Verification items for the finished model (mm, model axes). Face numbers are marked on the shaded views. Coordinates: 2 decimals unless noted, no trailing zeros. Order: outer loops, then holes, each group sorted by start corner. A loop starts at its lowest first (then second) coordinate and runs counter-clockwise, first axis right, second up. Notation, with made-up numbers: M 36.25,60 L 93.25,60 A14 ccw 93.25,64 Z; hole C 21.5,-32 d8. An arc over 180 degrees is marked long. Return JSON: item names as keys, results as strings. Group by question number.
Q1. Thickness scan on probe 1 along Y at (x, z) = (0, 68.75); probe 2 along Y at (x, z) = (0, 45.5); probe 3 along Z at (x, y) = (67.5, 74). Record the ranges inside material, lowest first.
Q2. Go/stop test with flat-tipped pins: pin 1 Ø1.5 at (x, z) = (71, 57) entering from +Y; pin 2 Ø0.9 at (y, z) = (-83.5, 5.5) entering from +X; pin 3 Ø10 at (y, z) = (-69, 57.5) entering from -X. Record where each tip stops, or that it passes through.
Q3. Mould release check, pull along Z, two halves, no side actions. Record for the marked faces 1, 2, 3 and 4: pulls with the +Z half, pulls with the -Z half, needs draft (parallel to the pull), parting line crosses it, or undercut.
Q4. Section check A-A, the plane y = 0. Enter the section's corners in (x, z), then the cut area to 3 significant figures.
Q5. Section check C-C, the plane x = -66.5. Enter the section's corners in (y, z).
Q6. Section check D-D, the plane y = 48. Enter the section's corners in (x, z).
from build123d import *

# Parameters (mm, degrees)
SKETCH1_R           = 100.8
SKETCH1_R_2         = 25.95
BOSS_EXTRUDE1_DEPTH = 4.84
SKETCH2_R           = 45.11
SKETCH2_R_2         = 25.95
BOSS_EXTRUDE2_DEPTH = 66.17
SKETCH3_R           = 100.8
SKETCH3_R_2         = 25.95
BOSS_EXTRUDE3_DEPTH = 4.84
SKETCH4_R           = 42.16
CUT_EXTRUDE1_DEPTH  = 15.86
BOSS_EXTRUDE4_START = 66.17
SKETCH5_R           = 95
SKETCH5_R_2         = 45.11
BOSS_EXTRUDE4_DEPTH = 66.17
SKETCH6_W           = 150
SKETCH6_H           = 1.75
BOSS_EXTRUDE5_DEPTH = 1.75
CUT_EXTRUDE5_DEPTH  = 90
SKETCH11_W          = 101.173290866
SKETCH11_H          = 1.75
CUT_EXTRUDE6_DEPTH  = 1.75


with BuildPart() as part:
    # Sketch1 → Boss-Extrude1 (new body)
    with BuildSketch(Plane.XY):
        with Locations(Location((0, 0, 0), (0, 0, 180))):
            Circle(SKETCH1_R)
        with Locations(Location((0, 0, 0), (0, 0, 180))):
            Circle(SKETCH1_R_2, mode=Mode.SUBTRACT)
    extrude(amount=BOSS_EXTRUDE1_DEPTH)

    # Sketch2 → Boss-Extrude2 (add)
    with BuildSketch(Plane.XY.offset(4.84)):
        Circle(SKETCH2_R)
        with Locations(Location((0, 0, 0), (0, 0, 180))):
            Circle(SKETCH2_R_2, mode=Mode.SUBTRACT)
    extrude(amount=BOSS_EXTRUDE2_DEPTH)

    # Sketch3 → Boss-Extrude3 (add)
    with BuildSketch(Plane.XY.offset(71.01)):
        with Locations(Location((0, 0, 0), (0, 0, 180))):
            Circle(SKETCH3_R)
        with Locations(Location((0, 0, 0), (0, 0, 180))):
            Circle(SKETCH3_R_2, mode=Mode.SUBTRACT)
    extrude(amount=BOSS_EXTRUDE3_DEPTH)

    # Sketch4 → Cut-Extrude1 (cut)
    with BuildSketch(Plane.XY.offset(75.85)):
        Circle(SKETCH4_R)
    extrude(amount=-CUT_EXTRUDE1_DEPTH, mode=Mode.SUBTRACT)

    # Sketch5 → Boss-Extrude4 (add)
    with BuildSketch(Plane(origin=(0, 0, 71.01), x_dir=(-1, 0, 0), z_dir=(0, 0, -1)).offset(BOSS_EXTRUDE4_START)):
        with Locations(Location((0, 0, 0), (0, 0, 180))):
            Circle(SKETCH5_R)
        Circle(SKETCH5_R_2, mode=Mode.SUBTRACT)
    boss_extrude4 = extrude(amount=-BOSS_EXTRUDE4_DEPTH)

    # Sketch6 → Boss-Extrude5 (add)
    with BuildSketch(Plane.XY.offset(4.84)):
        with Locations((75, -83.995)):
            Rectangle(SKETCH6_W, SKETCH6_H)
    boss_extrude5 = extrude(amount=BOSS_EXTRUDE5_DEPTH)

    # Sketch7 → Cut-Extrude5 (cut)
    with BuildSketch(Plane(origin=(150, 0, 0), x_dir=(0, 0, -1), z_dir=(1, 0, 0))):
        with BuildLine():
            Line((-6.333718434, -83.376281566), (-6.59, -83.12))
            Line((-6.59, -83.12), (-6.59, -83.995))
            ThreePointArc((-6.59, -83.995), (-6.523394591, -83.660151997), (-6.333718434, -83.376281566))
        make_face()
        with BuildLine():
            Line((-5.715, -83.12), (-6.59, -83.12))
            Line((-6.59, -83.12), (-6.333718434, -83.376281566))
            ThreePointArc((-6.333718434, -83.376281566), (-6.049848003, -83.186605409), (-5.715, -83.12))
        make_face()
        with BuildLine():
            Line((-4.84, -83.12), (-5.715, -83.12))
            ThreePointArc((-5.715, -83.12), (-5.096281566, -83.376281566), (-4.84, -83.995))
            Line((-4.84, -83.995), (-4.84, -83.12))
        make_face()
        with BuildLine():
            ThreePointArc((-4.84, -83.995), (-4.906605409, -84.329848003), (-5.096281566, -84.613718434))
            Line((-5.096281566, -84.613718434), (-4.84, -84.87))
            Line((-4.84, -84.87), (-4.84, -83.995))
        make_face()
        with BuildLine():
            Line((-4.84, -84.87), (-5.096281566, -84.613718434))
            ThreePointArc((-5.096281566, -84.613718434), (-5.380151997, -84.803394591), (-5.715, -84.87))
            Line((-5.715, -84.87), (-4.84, -84.87))
        make_face()
        with BuildLine():
            ThreePointArc((-5.715, -84.87), (-6.333718434, -84.613718434), (-6.59, -83.995))
            Line((-6.59, -83.995), (-6.59, -84.87))
            Line((-6.59, -84.87), (-5.715, -84.87))
        make_face()
    cut_extrude5 = extrude(amount=-CUT_EXTRUDE5_DEPTH, mode=Mode.SUBTRACT)

    # Mirror5: Boss-Extrude4, Boss-Extrude5, Cut-Extrude5 across plane
    add(boss_extrude4.mirror(Plane.ZX))
    add(boss_extrude5.mirror(Plane.ZX))
    add(cut_extrude5.mirror(Plane.ZX), mode=Mode.SUBTRACT)

    # Sketch11 → Cut-Extrude6 (cut)
    with BuildSketch(Plane.XZ.offset(84.87)):
        with Locations((99.413354567, 5.715)):
            Rectangle(SKETCH11_W, SKETCH11_H)
    extrude(amount=-CUT_EXTRUDE6_DEPTH, mode=Mode.SUBTRACT)


solid = part.part
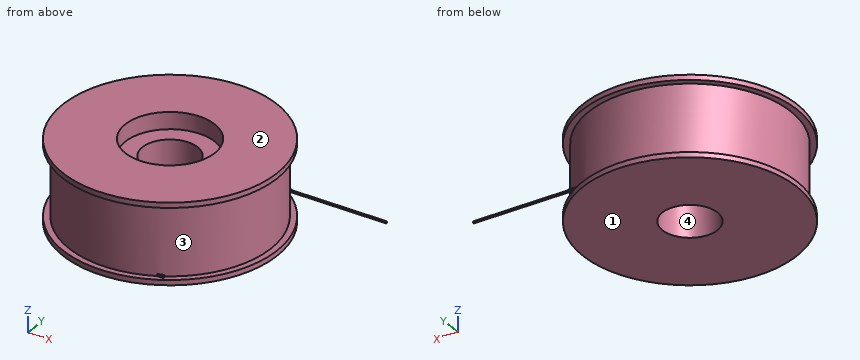
Numbers:
{
 "1": {"probe 1": "y = -95 to -42.16, 42.16 to 95", "probe 2": "y = -95 to -25.95, 25.95 to 95", "probe 3": "z = 0 to 4.84, 71.01 to 75.85"},
 "2": {"pin 1": "stops at y = 63.95", "pin 2": "stops at x = 48.83", "pin 3": "stops at x = -70.21"},
 "3": {"face 1": "pulls with the -Z half", "face 2": "pulls with the +Z half", "face 3": "undercut", "face 4": "needs draft"},
 "4": {"outline": "M -100.8,0 L -25.95,0 L -25.95,59.99 L -42.16,59.99 L -42.16,75.85 L -100.8,75.85 L -100.8,71.01 L -95,71.01 L -95,4.84 L -100.8,4.84 Z; M 25.95,0 L 100.8,0 L 100.8,4.84 L 95,4.84 L 95,71.01 L 100.8,71.01 L 100.8,75.85 L 42.16,75.85 L 42.16,59.99 L 25.95,59.99 Z", "area": "10,100 mm2"},
 "5": {"outline": "M -75.75,0 L 75.75,0 L 75.75,4.84 L 67.84,4.84 L 67.84,71.01 L 75.75,71.01 L 75.75,75.85 L -75.75,75.85 L -75.75,71.01 L -67.84,71.01 L -67.84,4.84 L -75.75,4.84 Z"},
 "6": {"outline": "M -88.64,0 L 88.64,0 L 88.64,4.84 L 81.98,4.84 L 81.98,71.01 L 88.64,71.01 L 88.64,75.85 L -88.64,75.85 L -88.64,71.01 L -81.98,71.01 L -81.98,4.84 L -88.64,4.84 Z"}
}
